from build123d import *

# Parameters (mm, degrees)
SKETCH_1_W          = 34
SKETCH_1_H          = 87
SKETCH_1_R          = 0.6
EXTRUDE_1_DEPTH     = 4
SKETCH_2_W          = 22
SKETCH_2_H          = 3
SKETCH_2_W_2        = 3
SKETCH_2_H_2        = 75
SKETCH_2_W_3        = 16
SKETCH_2_H_3        = 21
SKETCH_2_R          = 1.25
SKETCH_2_H_4        = 12
SKETCH_2_H_5        = 24
CUT_EXTRUDE_1_DEPTH = 94.493315269
SKETCH_3_R          = 1.75
CUT_EXTRUDE_2_DEPTH = 2


with BuildPart() as part:
    # 草图1 → 凸台-拉伸1 (new body)
    with BuildSketch(Plane(origin=(0, 0, 0), x_dir=(1, 0, 0), z_dir=(0, 1, 0))):
        with Locations((17, -43.5)):
            Rectangle(SKETCH_1_W, SKETCH_1_H)
        with Locations(Location((3, -3, 0), (0, 0, 270))):
            Circle(SKETCH_1_R, mode=Mode.SUBTRACT)
        with Locations(Location((31, -3, 0), (0, 0, 270))):
            Circle(SKETCH_1_R, mode=Mode.SUBTRACT)
        with Locations(Location((31, -84, 0), (0, 0, 270))):
            Circle(SKETCH_1_R, mode=Mode.SUBTRACT)
        with Locations(Location((3, -84, 0), (0, 0, 270))):
            Circle(SKETCH_1_R, mode=Mode.SUBTRACT)
    extrude(amount=EXTRUDE_1_DEPTH)

    # 草图2 → 切除-拉伸1 (cut, through all)
    with BuildSketch(Plane(origin=(0, 4, 0), x_dir=(1, 0, 0), z_dir=(0, 1, 0))):
        with Locations((17, -1.5)):
            Rectangle(SKETCH_2_W, SKETCH_2_H)
        with Locations((1.5, -43.5)):
            Rectangle(SKETCH_2_W_2, SKETCH_2_H_2)
        with Locations((32.5, -43.5)):
            Rectangle(SKETCH_2_W_2, SKETCH_2_H_2)
        with Locations((17, -85.5)):
            Rectangle(SKETCH_2_W, SKETCH_2_H)
        with Locations((17, -19.5)):
            Rectangle(SKETCH_2_W_3, SKETCH_2_H_3)
        with Locations(Location((17, -33, 0), (0, 0, 270))):
            Circle(SKETCH_2_R)
        with Locations((17, -72)):
            Rectangle(SKETCH_2_W_3, SKETCH_2_H_4)
        with Locations(Location((17, -63, 0), (0, 0, 270))):
            Circle(SKETCH_2_R)
        with Locations((17, -48)):
            Rectangle(SKETCH_2_W_3, SKETCH_2_H_5)
    extrude(amount=-CUT_EXTRUDE_1_DEPTH, mode=Mode.SUBTRACT)

    # 草图3 → 切除-拉伸2 (cut)
    with BuildSketch(Plane.XZ):
        with Locations(Location((17, 63, 0), (0, 0, 270))):
            Circle(SKETCH_3_R)
        with Locations(Location((17, 33, 0), (0, 0, 270))):
            Circle(SKETCH_3_R)
    extrude(amount=-CUT_EXTRUDE_2_DEPTH, mode=Mode.SUBTRACT)


solid = part.part
Geometry check sheet. Reference: the model listing, model coordinates, mm. A direction names the side the tool comes from. Round coordinates to 2 decimals unless told otherwise and drop trailing zeros. Loops run counter-clockwise (first coordinate to the right, second up) from the corner with the lowest first, then second, coordinate; pieces in that order, holes last. Notation, with made-up numbers: (-33.75, -1) - (18.25, -1) arc R27 cw to (18.25, 20) - close; hole circle Ø2 at (6.25, 79.25). An arc over 180 degrees is marked (long way). One line per question, with ' | ' between items. Start each with the question number.
1. Depth check by flat-ended pin: pin 1 (2 mm diameter, centred on x = 17, z = 63, fed in from -Y); pin 2 (2 mm diameter, centred on y = 3, z = 14.5, fed in from +X); pin 3 (1.2 mm diameter, centred on x = 16, y = 2, fed in from +Z); pin 4 (3 mm diameter, centred on x = 17, z = 33, fed in from -Y). Enter the tip coordinate at first touch or a pass-through.
2. Cross-section at D-D on z = 33. Record the cut outline in (x, y), then the cut area to 3 significant figures.
3. Scan lines: line 1 (Z direction, x = 19, y = 0.5); line 2 (X direction, y = 1.25, z = 47); line 3 (Z direction, x = 32, y = 0.7). Record each from-to range of solid material in increasing order. Write a range as [from, to].
4. Cross-section at A-A on x = 20.5. Record the cut outline in (y, z).
5. Cross-section at B-B on z = 11.5. Record the cut outline in (x, y).
6. Cross-section at C-C on x = 17. State how many separate pieces and enclosed holes the cut face has, then the cut area to 3 significant figures.
7. Tool access check on faces 5 (the face through (17, 2, 60)), 6 (the face through (3, 2, 87)), 7 (the face through (17, 2, 84)), 8 (the face through (1, 2, 81)), 9 (the face through (17.526, 0.986, 61.331)). Record the directions out of +Z, -Z, +X, -X, +Y, -Y that give a thin tool (end or side, any length) a straight path to the whole face; none if there is none.
8. Draft check along Z on faces 1 (the face through (31, 2, 87)), 2 (the face through (18.18, 0.99, 34.29)), 3 (the face through (6, 2, 2)), 4 (the face through (17.38, 3.01, 64.19)). Enter one of: released by +Z, released by -Z, zero draft, split by the parting line, or undercut.
Taken from the geometry:
1) pin 1: through | pin 2: x = 31 | pin 3: z = 84 | pin 4: y = 2
2) outline: (3, 0) - (15.25, 0) - (15.25, 2) - (15.75, 2) - (15.75, 4) - (3, 4) - close; (18.25, 2) - (18.75, 2) - (18.75, 0) - (31, 0) - (31, 4) - (18.25, 4) - close | area: 100 mm²
3) line 1: [3, 9], [30, 36], [60, 66], [78, 84] | line 2: [3, 9], [25, 31] | line 3: [0, 6], [81, 87]
4) outline: (0, 3) - (4, 3) - (4, 9) - (0, 9) - close; (0, 30) - (4, 30) - (4, 36) - (0, 36) - close; (0, 60) - (4, 60) - (4, 66) - (0, 66) - close; (0, 78) - (4, 78) - (4, 84) - (0, 84) - close
5) outline: (3, 0) - (9, 0) - (9, 4) - (3, 4) - close; (25, 0) - (31, 0) - (31, 4) - (25, 4) - close
6) separate pieces: 6 | enclosed holes: 0 | area: 72.0 mm²
7) face 5: +Y, -Y | face 6: +Z, +X, -X, +Y, -Y | face 7: +Z, +Y, -Y | face 8: -X, +Y, -Y | face 9: -Y
8) face 1: released by +Z | face 2: undercut | face 3: zero draft | face 4: undercut
